Model file for the job. Use its own axes, mm. Round coordinates to 2 decimals unless told otherwise and drop trailing zeros. Loops run counter-clockwise (first coordinate to the right, second up) from the corner with the lowest first, then second, coordinate; pieces in that order, holes last. Notation, with made-up numbers: (85, 89.5) -> (125, 89.5) arc R21 cw to (125, 115.5) -> close; hole circle Ø6 at (-39.75, 36.5). An arc over 180 degrees is marked (long way). Use a Markdown table: item, result.
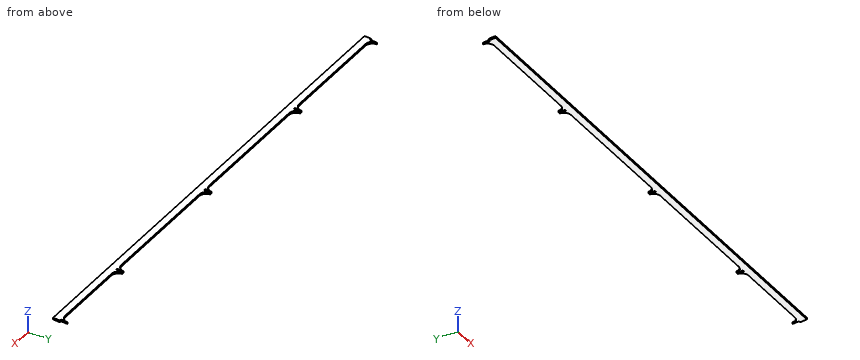
from build123d import *

# Parameters (mm, degrees)
EXTRUDE_1_DEPTH = 2


with BuildPart() as part:
    # Model → 凸台-拉伸1 (new body)
    with BuildSketch(Plane.XY):
        with BuildLine():
            Line((5.143788589, 18.04241923), (4.137613793, 9.847783121))
            Line((4.137613793, 9.847783121), (580.873096163, 12.99559552))
            Line((580.873096163, 12.99559552), (581.848050911, 20.935964733))
            Line((581.848050911, 20.935964733), (579.866676478, 21.179246923))
            Line((579.866676478, 21.179246923), (580.791756024, 28.713415216))
            ThreePointArc((580.791756024, 28.713415216), (577.819958349, 23.132995179), (571.91207976, 20.881409119))
            Line((571.91207976, 20.881409119), (485.690224553, 20.411136961))
            ThreePointArc((485.690224553, 20.411136961), (480.53763707, 22.90043185), (478.665298456, 28.307842962))
            Line((478.665298456, 28.307842962), (477.690343709, 20.367473749))
            Line((477.690343709, 20.367473749), (475.708969276, 20.610755938))
            Line((475.708969276, 20.610755938), (476.634048822, 28.144924232))
            ThreePointArc((476.634048822, 28.144924232), (473.633509712, 22.539262149), (467.677868383, 20.31282583))
            Line((467.677868383, 20.31282583), (322.805939428, 19.522117319))
            ThreePointArc((322.805939428, 19.522117319), (317.653351945, 22.011412208), (315.781013331, 27.418823319))
            Line((315.781013331, 27.418823319), (314.806058584, 19.478454106))
            Line((314.806058584, 19.478454106), (312.824684151, 19.721736296))
            Line((312.824684151, 19.721736296), (313.749763697, 27.25590459))
            ThreePointArc((313.749763697, 27.25590459), (310.749224588, 21.650242507), (304.793583258, 19.423806187))
            Line((304.793583258, 19.423806187), (156.683570496, 18.615424271))
            ThreePointArc((156.683570496, 18.615424271), (151.530983012, 21.104719159), (149.658644399, 26.512130271))
            Line((149.658644399, 26.512130271), (148.683689651, 18.571761058))
            Line((148.683689651, 18.571761058), (146.702315218, 18.815043248))
            Line((146.702315218, 18.815043248), (147.627394764, 26.349211541))
            ThreePointArc((147.627394764, 26.349211541), (144.626855655, 20.743549458), (138.671214325, 18.517113139))
            Line((138.671214325, 18.517113139), (15.125043867, 17.842800254))
            ThreePointArc((15.125043867, 17.842800254), (9.972456383, 20.332095142), (8.10011777, 25.739506254))
            Line((8.10011777, 25.739506254), (7.125163022, 17.799137041))
            Line((7.125163022, 17.799137041), (5.143788589, 18.04241923))
        make_face()
    extrude(amount=EXTRUDE_1_DEPTH)


solid = part.part
Q1. Band-saw the part on A-A, the plane z = 0.8. Give the cut face in (x, y).
Results list:
| item | result |
|---|---|
| outline | (4.14, 9.85) -> (580.87, 13) -> (581.85, 20.94) -> (579.87, 21.18) -> (580.79, 28.71) arc R9.01 cw to (571.91, 20.88) -> (485.69, 20.41) arc R7.46 cw to (478.67, 28.31) -> (477.69, 20.37) -> (475.71, 20.61) -> (476.63, 28.14) arc R9.01 cw to (467.68, 20.31) -> (322.81, 19.52) arc R7.46 cw to (315.78, 27.42) -> (314.81, 19.48) -> (312.82, 19.72) -> (313.75, 27.26) arc R9.01 cw to (304.79, 19.42) -> (156.68, 18.62) arc R7.46 cw to (149.66, 26.51) -> (148.68, 18.57) -> (146.7, 18.82) -> (147.63, 26.35) arc R9.01 cw to (138.67, 18.52) -> (15.13, 17.84) arc R7.46 cw to (8.1, 25.74) -> (7.13, 17.8) -> (5.14, 18.04) -> close |
Q2. Drill centre lines: L1, parallel to Y at x = 211, z = 0.55; L2, parallel to Y at x = 286, z = 1.75; L3, parallel to X at y = 13.75, z = 1.75. Where is each one in solid material? Low to high. Write a range as from..to.
Results list:
| item | result |
|---|---|
| L1 | y = 10.98..18.91 |
| L2 | y = 11.39..19.32 |
| L3 | x = 4.62..580.97 |
Q3. Flat gauge pin, fed straight in: pin 1 (1 mm diameter, centred on y = 19.5, z = 1.5, fed in from -X). Where does the tip first touch, or does it go through?
Results list:
| item | result |
|---|---|
| pin 1 | stops at x = 7.27 |
Q4. Band-saw the part on B-B, the plane x = 71. Give the cut face in (y, z).
Results list:
| item | result |
|---|---|
| outline | (10.21, 0) -> (18.15, 0) -> (18.15, 2) -> (10.21, 2) -> close |
